CAD build for the part. Positions are in the model's coordinates, mm. A direction names the side the tool comes from. Round coordinates to 2 decimals unless told otherwise and drop trailing zeros. Order: outer loops, then holes, each group sorted by start corner. A loop starts at its lowest first (then second) coordinate and runs counter-clockwise, first axis right, second up.
Autodesk Fusion 360 part; units mm, degrees
sketch "Sketch1" plane through (0, 0, 0) normal (0, 1, 0) x (1, 0, 0)
  circle A0 centre (0, 0) radius 3
  dimension "d1" = 6
extrude "Extrude1" add sketch "Sketch1" along normal blind 13
sketch "Sketch2" plane through (0, 0, 0) normal (0, -1, 0) x (1, 0, 0)
  circle A0 centre (0, 0) radius 3
  circle A1 centre (0, 0) radius 9
  dimension "d4" = 18
extrude "Extrude2" add sketch "Sketch2" along normal blind 7 contours A0 | A1
sketch "Sketch3" plane through (0, -7, 0) normal (0, -1, 0) x (1, 0, 0)
  circle A0 centre (0, 0) radius 9
  circle A1 centre (0, 0) radius 6.4
  dimension "d7" = 12.8
extrude "Extrude3" cut sketch "Sketch3" against normal blind 5 contours A1
sketch "Sketch4" plane through (0, -2, 0) normal (0, -1, 0) x (1, 0, 0)
  circle A0 centre (0, 0) radius 6.4
  circle A1 centre (0, 0) radius 2
  dimension "d10" = 4
hole "Hole1" at (0, -2, 0) direction (0, 1, 0) diameter 3.332 depth 5 tip angle 118
chamfer "Chamfer1" distance 3 angle 45 1 edges at (-2.797, 0, 1.0848)
extrude "Extrude4" add 1 faces at (0.3505, 13, 0.866) along direction (0, 1, 0) blind 2
1. Cut at B-B, the plane y = 2.5. Write the cut outline in (x, z), and give its area (3 significant figures).
2. Cut at A-A, the plane y = 7. Write the cut outline in (x, z).
3. Mould opens along X. For faces 4 (the face through (-5.08, -4.54, -3.89)), 5 (the face through (0, 15, 0)), 6 (the face through (-3, 9, 0)) say: released by +X, released by -X, zero draft, split by the parting line, or undercut.
4. Tool access for faces 1 (the face through (2, 0, -6)), 2 (the face through (4, -7, -6)), 3 (the face through (1.3, -2, -1.3)): list every direction of +Z, -Z, +X, -X, +Y, -Y with a clear straight run to the whole face (end or side of a thin tool).
5. Cut at C-C, the plane z = -7.5. Write the cut outline in (x, y).
6. Pin check, flat tips, straight feed: P1, Ø4, axis at x = -2, z = 1.5, coming from the -Y side; P2, Ø1.5, axis at y = -3.5, z = -4, coming from the +X side. Stop position of each tip, or through.
7. Drill centre lines: line 1 (Z direction, x = 0, y = -5.9); line 2 (Y direction, x = 6.25, z = -5.25); line 3 (Y direction, x = 2.75, z = 1). Where is each one in solid material? Low to high.
Outcome:
1. outline: circle Ø7 at (0, 0); hole circle Ø3.33 at (0, 0)
1. area: 29.8 mm2
2. outline: circle Ø6 at (0, 0)
3. face 4: undercut
3. face 5: zero draft
3. face 6: split by the parting line
4. face 1: +Y
4. face 2: +Z, -Z, +X, -X, -Y
4. face 3: -Y
5. outline: (-4.97, -7) - (4.97, -7) - (4.97, 0) - (-4.97, 0) - close
6. P1: stops at y = -2
6. P2: stops at x = 8.39
7. line 1: z = -9 to -6.4, 6.4 to 9
7. line 2: y = -7 to 0
7. line 3: y = -2 to 15
